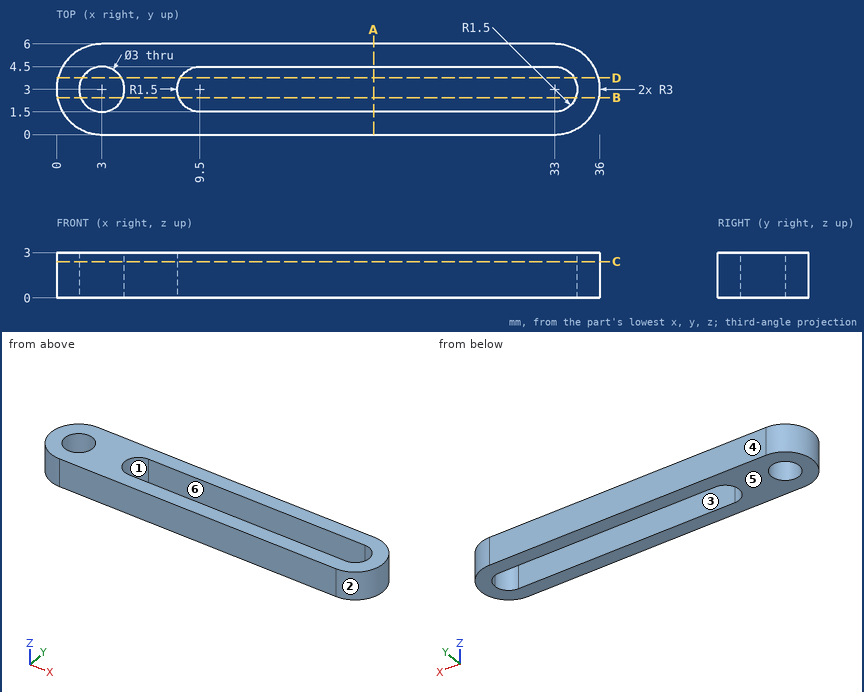
Here's the drawing with two shaded views (mm, measured from the low corner). I have some questions. A direction names the side the tool comes from. Give positions to 0.01 mm unless a question says otherwise; leave off trailing zeros. Loops run counter-clockwise (first coordinate to the right, second up) from the corner with the lowest first, then second, coordinate; pieces in that order, holes last. Notation, with made-up numbers: M 54,-35 L 72,-35 A14 cw 72,-15 Z; hole C 44.5,68.25 d2. An arc over 180 degrees is marked long. Use one line per item in the form item = value. Start each with the question number.
Q1. Thinking about a two-plate mould opening in Y: for the marked faces 1, 2, 3 and 4, which applies, +Y half, -Y half, draft (parallel to the pull), parting line (faces both ways), or undercut?
Q2. I need wall thicknesses on line 1 along Y through (x, z) = (3, 1.7); line 2 along X through (y, z) = (1.9, 1.75); line 3 along X through (y, z) = (1.8, 0.4). Which ranges of each line are inside material? Lowest first, please.
Q3. Which directions (+Z, -Z, +X, -X, +Y, -Y) give clear straight access to the entire face, cutting with the end or side of a thin tool? Please do the marked faces 5 and 6.
Q4. If we section it at B-B (y = 2.45): Write out the boundary of the cut face in (x, z), then the cut area to 3 significant figures.
Q5. If we section it at D-D (y = 3.75): Write out the boundary of the cut face in (x, z).
Q6. If we section it at C-C (z = 2.4): Write out the boundary of the cut face in (x, y), then the cut area to 3 significant figures.
Q7. If we section it at A-A (x = 21): Write out the boundary of the cut face in (y, z).
Q8. Will this pin go through, and if not, where does the flat tip stop? pin 1 Ø1.5 at (y, z) = (4.5, 1.5) entering from -X.
Taken from the geometry:
q1.face_1 = undercut
q1.face_2 = parting line
q1.face_3 = undercut
q1.face_4 = +Y half
q2.line_1 = 0 to 1.5, 4.5 to 6
q2.line_2 = 0.21 to 1.98, 4.02 to 8.48, 34.02 to 35.79
q2.line_3 = 0.25 to 2.1, 3.9 to 8.6, 33.9 to 35.75
q3.face_5 = -Z, +X, -X, +Y, -Y
q3.face_6 = +Z, -Z
q4.outline = M 0.05,0 L 1.6,0 L 1.6,3 L 0.05,3 Z; M 4.4,0 L 8.1,0 L 8.1,3 L 4.4,3 Z; M 34.4,0 L 35.95,0 L 35.95,3 L 34.4,3 Z
q4.area = 20.4 mm^2
q5.outline = M 0.1,0 L 1.7,0 L 1.7,3 L 0.1,3 Z; M 4.3,0 L 8.2,0 L 8.2,3 L 4.3,3 Z; M 34.3,0 L 35.9,0 L 35.9,3 L 34.3,3 Z
q6.outline = M 3,0 L 33,0 A3 ccw 33,6 L 3,6 A3 ccw Z; hole C 3,3 d3; hole M 9.5,1.5 L 33,1.5 A1.5 ccw 34.5,3 A1.5 ccw 33,4.5 L 9.5,4.5 A1.5 ccw Z
q6.area = 124 mm^2
q7.outline = M 0,0 L 1.5,0 L 1.5,3 L 0,3 Z; M 4.5,0 L 6,0 L 6,3 L 4.5,3 Z
q8.pin_1 = 0.1
